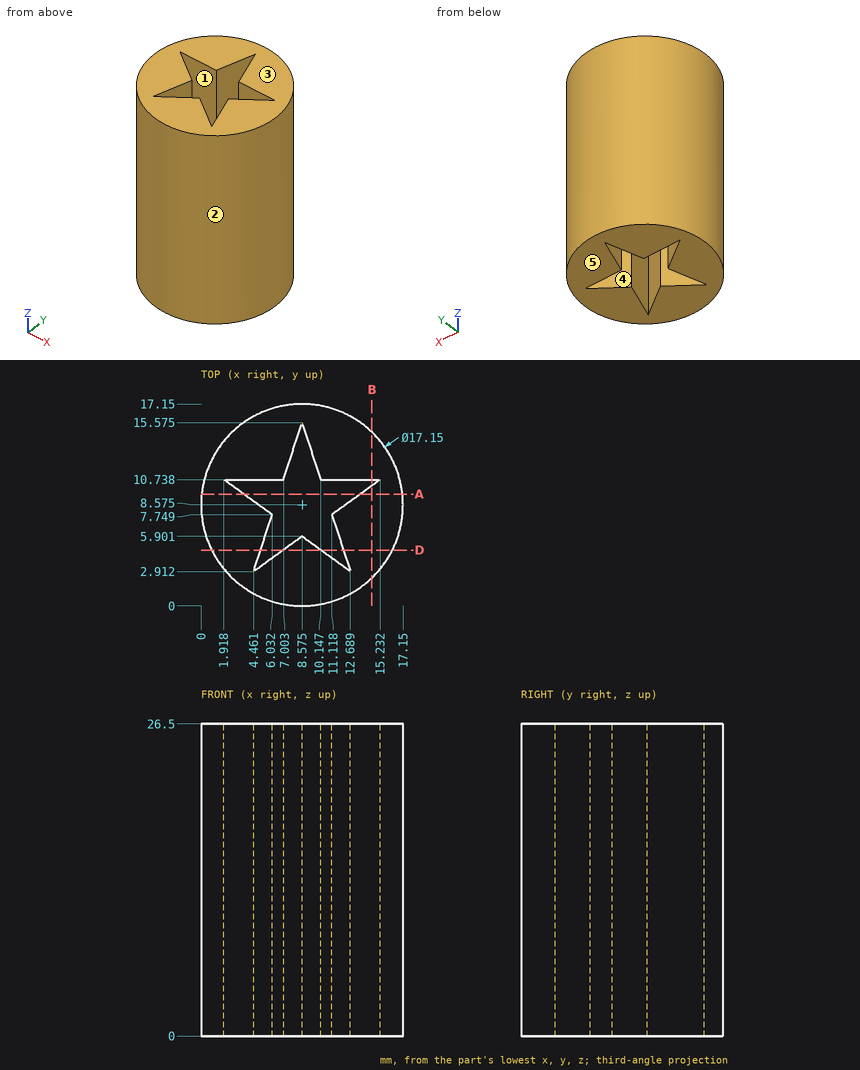
Geometry check sheet. Reference: drawing and pictorial views, mm from the part's lowest x, y, z. A direction names the side the tool comes from. Give positions to 0.01 mm unless a question says otherwise; leave off trailing zeros. Order: outer loops, then holes, each group sorted by start corner. A loop starts at its lowest first (then second) coordinate and runs counter-clockwise, first axis right, second up. Notation, with made-up numbers: (13.5, 23) -> (40.5, 23) arc R11 ccw to (40.5, 30) -> close; hole circle Ø8 at (27.5, 52). An arc over 180 degrees is marked (long way). Write each question's results on one line, items separated by ' | '. Start each with the question number.
(1) Scan lines: line 1 (X direction, y = 5.25, z = 9.5) (1 decimal); line 2 (X direction, y = 3.25, z = 23.75) (1 decimal); line 3 (X direction, y = 6.5, z = 9.5) (1 decimal). Record each from-to range of solid material in increasing order.
(2) Sectioned sample at A-A (y = 9.5). Enter the section's corners in (x, z), plus the area to 3 significant figures.
(3) Sectioned sample at B-B (x = 14.5). Enter the section's corners in (y, z) (1 decimal).
(4) Gauge pin test, flat ends, axial feed: P1, Ø4, axis at x = 11.5, z = 15, coming from the -Y side; P2, Ø2, axis at y = 2, z = 11, coming from the +X side; P3, Ø6, axis at y = 5, z = 21, coming from the -X side. Record the tip position at first contact, or that the pin passes through.
(5) Sectioned sample at D-D (y = 4.75). Enter the section's corners in (x, z).
(6) Mould release check, pull along Y, two halves, no side actions. Record for the marked faces 1, 2 and 3: pulls with the +Y half, pulls with the -Y half, needs draft (parallel to the pull), parting line crosses it, or undercut.
(7) Access from +Z, -Z, +X, -X, +Y, -Y to the whole of each face (thin tool, end or side, straight path). Record for the marked faces 4 and 5.
Answer below:
1) line 1: 0.7 to 5.2, 7.7 to 9.5, 11.9 to 16.5 | line 2: 1.9 to 4.6, 4.9 to 12.2, 12.6 to 15.3 | line 3: 0.3 to 5.6, 11.5 to 16.9
2) outline: (0.05, 0) -> (3.62, 0) -> (3.62, 26.5) -> (0.05, 26.5) -> close; (13.53, 0) -> (17.1, 0) -> (17.1, 26.5) -> (13.53, 26.5) -> close | area: 189 mm2
3) outline: (2.4, 0) -> (10.2, 0) -> (10.2, 26.5) -> (2.4, 26.5) -> close; (10.7, 0) -> (14.8, 0) -> (14.8, 26.5) -> (10.7, 26.5) -> close
4) P1: y = 0.05 | P2: x = 15.09 | P3: x = 0.02
5) outline: (0.9, 0) -> (5.06, 0) -> (5.06, 26.5) -> (0.9, 26.5) -> close; (6.99, 0) -> (10.16, 0) -> (10.16, 26.5) -> (6.99, 26.5) -> close; (12.09, 0) -> (16.25, 0) -> (16.25, 26.5) -> (12.09, 26.5) -> close
6) face 1: undercut | face 2: parting line crosses it | face 3: needs draft
7) face 4: +Z, -Z | face 5: -Z, +X, -X, +Y, -Y
